For this review, take the finished solid that the model builds, in its own axes (mm). Face numbers are marked on the shaded views. A direction names the side the tool comes from. Round coordinates to 2 decimals unless told otherwise and drop trailing zeros. Order: outer loops, then holes, each group sorted by start corner. A loop starts at its lowest first (then second) coordinate and runs counter-clockwise, first axis right, second up. Notation, with made-up numbers: (38.25, 60.25) - (88.25, 60.25) arc R20 cw to (88.25, 74.25) - close; hole circle Ø11 at (59.25, -28). An arc over 180 degrees is marked (long way). One line per question, with ' | ' between items.
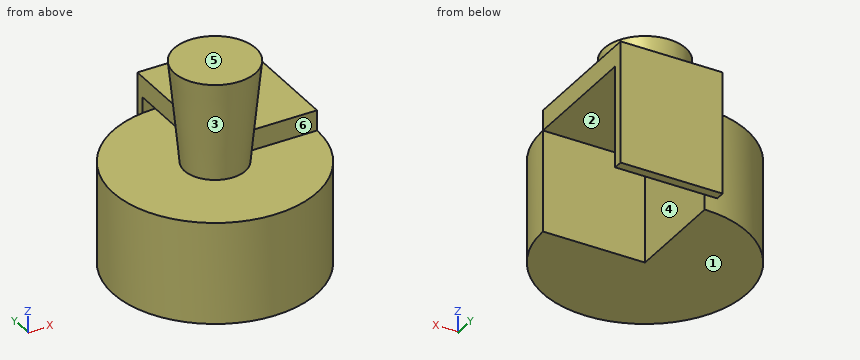
```python
from build123d import *

# Parameters (mm, degrees)
CYLINDER_R     = 10
CYLINDER_DEPTH = 10
BOX_W          = 10
BOX_H          = 13
BOX_DEPTH      = 12
BOX001_W       = 10.1
BOX001_H       = 12.1
BOX001_DEPTH   = 10


with BuildPart() as part:
    # Cone → Cone (revolve)
    with BuildSketch(Plane.XZ):
        Polygon((0, 0), (2, 0), (4, 20), (0, 20), align=None)
    revolve(axis=Axis((0, 0, 0), (0, 0, 1)))

    # Cylinder → Cylinder (join)
    with BuildSketch(Plane.XY):
        Circle(CYLINDER_R)
    extrude(amount=CYLINDER_DEPTH)

    # Box → Box (join)
    with BuildSketch(Plane.XY):
        with Locations((5, 6.5)):
            Rectangle(BOX_W, BOX_H)
    extrude(amount=BOX_DEPTH)

    # Box001 → Box001 (cut)
    with BuildSketch(Plane.XY):
        with Locations((5.05, 6.05)):
            Rectangle(BOX001_W, BOX001_H)
    extrude(amount=BOX001_DEPTH, mode=Mode.SUBTRACT)


solid = part.part
```
(1) We need section C-C on z = 13.5. State the section outline as (x, y) points, plus the area to 3 significant figures.
Output values:
outline: circle Ø6.7 at (0, 0) | area: 35.3 mm^2
(2) Insertion check: pin 1 (5 mm diameter, centred on y = 8, z = 8.5, fed in from -X); pin 2 (3 mm diameter, centred on x = 6, z = 3, fed in from -Y); pin 3 (1 mm diameter, centred on y = 3, z = 14, fed in from -X). Each pin has a flat end and moves straight along its axis. Give the tip position at first contact, or say it passes through.
Output values:
pin 1: x = -8.35 | pin 2: y = -8.93 | pin 3: x = -2.31
(3) Mouldability with a two-part tool opening along Y and no side actions: class the marked faces 4, 5 and 6 as released by +Y, released by -Y, zero draft, split by the parting line, or undercut.
Output values:
face 4: undercut | face 5: zero draft | face 6: released by -Y
(4) For the marked faces 1, 2 and 3, list the 3-axis set-ups (+Z, -Z, +X, -X, +Y, -Y) from which the entire face can be reached by the end or side of a thin tool; tool diameter is ignored.
Output values:
face 1: -Z, +X, -X, +Y, -Y | face 2: -Z, +X | face 3: none
(5) For probe 1 along Z at (x, y) = (2.25, 4.75); probe 2 along Z at (x, y) = (-7.5, 4.75); probe 3 along Y at (x, z) = (7.5, 6.75), list the stretches that pass through material, from the lowest coordinate up. Write a range as [from, to].
Output values:
probe 1: [10, 12] | probe 2: [0, 10] | probe 3: [-6.61, 0], [12.1, 13]
(6) We need section D-D on y = -6. State the section outline as (x, z) points, plus the area to 3 significant figures.
Output values:
outline: (-8, 0) - (8, 0) - (8, 10) - (-8, 10) - close | area: 160 mm^2
(7) We need section A-A on z = 8.75. State the section outline as (x, y) points.
Output values:
outline: (0, 0) - (0, 10) arc R10 ccw (long way) to (10, 0) - close; (0, 12.1) - (10, 12.1) - (10, 13) - (0, 13) - close
